Source: CAD feature listing. Evaluate the final solid. Frame: model axes, mm. Face numbers are marked on the shaded views. A direction names the side the tool comes from. Coordinates: 2 decimals unless noted, no trailing zeros. Order: outer loops, then holes, each group sorted by start corner. A loop starts at its lowest first (then second) coordinate and runs counter-clockwise, first axis right, second up.
```python
from build123d import *

# Parameters (mm, degrees)
BOSS_EXTRUDE1_START     = -9
SKETCH1_W               = 152.45
SKETCH1_H               = 16
BOSS_EXTRUDE1_DEPTH     = 5
BOSS_EXTRUDE2_START     = -9
SKETCH2_R               = 6.5
BOSS_EXTRUDE2_DEPTH     = 5
BOSS_EXTRUDE3_START     = -9
SKETCH3_R               = 8
BOSS_EXTRUDE3_DEPTH     = 5
BOSS_EXTRUDE4_START     = -9
SKETCH4_R               = 7
BOSS_EXTRUDE4_DEPTH     = 11.5
BOSS_EXTRUDE5_START     = 2.5
SKETCH5_R               = 5.5
BOSS_EXTRUDE5_DEPTH     = 1
BOSS_EXTRUDE6_START     = -4
SKETCH6_R               = 3.5
BOSS_EXTRUDE6_DEPTH     = 1
CUT_EXTRUDE1_DEPTH      = 132.004589614
CUT_EXTRUDE1_DEPTH_BACK = 132.004589614
SKETCH7_R               = 4
CUT_EXTRUDE2_DEPTH      = 132.004589614
CUT_EXTRUDE2_DEPTH_BACK = 132.004589614
SKETCH8_R               = 1.725
CUT_EXTRUDE3_DEPTH      = 132.004589614
CUT_EXTRUDE3_DEPTH_BACK = 132.004589614
SKETCH9_W               = 22.8
SKETCH9_H               = 11.9
CUT_EXTRUDE4_DEPTH      = 132.004589614
CUT_EXTRUDE4_DEPTH_BACK = 132.004589614
SKETCH10_R              = 0.9


with BuildPart() as part:
    # Sketch1 → Boss-Extrude1 (new body)
    with BuildSketch(Plane.XY.offset(BOSS_EXTRUDE1_START)):
        with Locations((46.225, 0)):
            Rectangle(SKETCH1_W, SKETCH1_H)
    extrude(amount=BOSS_EXTRUDE1_DEPTH)

    # Sketch2 → Boss-Extrude2 (add)
    with BuildSketch(Plane.XY.offset(BOSS_EXTRUDE2_START)):
        with Locations((-30, 0)):
            Circle(SKETCH2_R)
    extrude(amount=BOSS_EXTRUDE2_DEPTH)

    # Sketch3 → Boss-Extrude3 (add)
    with BuildSketch(Plane.XY.offset(BOSS_EXTRUDE3_START)):
        with Locations((122.45, 0)):
            Circle(SKETCH3_R)
    extrude(amount=BOSS_EXTRUDE3_DEPTH)

    # Sketch4 → Boss-Extrude4 (add)
    with BuildSketch(Plane.XY.offset(BOSS_EXTRUDE4_START)):
        Circle(SKETCH4_R)
    extrude(amount=BOSS_EXTRUDE4_DEPTH)

    # Sketch5 → Boss-Extrude5 (add)
    with BuildSketch(Plane.XY.offset(BOSS_EXTRUDE5_START)):
        Circle(SKETCH5_R)
    extrude(amount=BOSS_EXTRUDE5_DEPTH)

    # Sketch6 → Boss-Extrude6 (add)
    with BuildSketch(Plane.XY.offset(BOSS_EXTRUDE6_START)):
        with Locations((-30, 0)):
            Circle(SKETCH6_R)
    extrude(amount=BOSS_EXTRUDE6_DEPTH)

    # Sketch7 → Cut-Extrude1 (cut, two sides: drawn at the far end of the back side and taken through both)
    with BuildSketch(Plane.XY.offset(-CUT_EXTRUDE1_DEPTH_BACK)):
        Circle(SKETCH7_R)
    extrude(amount=CUT_EXTRUDE1_DEPTH + CUT_EXTRUDE1_DEPTH_BACK, mode=Mode.SUBTRACT)

    # Sketch8 → Cut-Extrude2 (cut, two sides: drawn at the far end of the back side and taken through both)
    with BuildSketch(Plane.XY.offset(-CUT_EXTRUDE2_DEPTH_BACK)):
        with Locations((-30, 0)):
            Circle(SKETCH8_R)
    extrude(amount=CUT_EXTRUDE2_DEPTH + CUT_EXTRUDE2_DEPTH_BACK, mode=Mode.SUBTRACT)

    # Sketch9 → Cut-Extrude3 (cut, two sides: drawn at the far end of the back side and taken through both)
    with BuildSketch(Plane.XY.offset(-CUT_EXTRUDE3_DEPTH_BACK)):
        with Locations((114.2, 0)):
            Rectangle(SKETCH9_W, SKETCH9_H)
    extrude(amount=CUT_EXTRUDE3_DEPTH + CUT_EXTRUDE3_DEPTH_BACK, mode=Mode.SUBTRACT)

    # Sketch10 → Cut-Extrude4 (cut, two sides: drawn at the far end of the back side and taken through both)
    with BuildSketch(Plane.XY.offset(-CUT_EXTRUDE4_DEPTH_BACK)):
        with Locations((100.45, 0)):
            Circle(SKETCH10_R)
        with Locations((127.95, 0)):
            Circle(SKETCH10_R)
    extrude(amount=CUT_EXTRUDE4_DEPTH + CUT_EXTRUDE4_DEPTH_BACK, mode=Mode.SUBTRACT)


solid = part.part
```
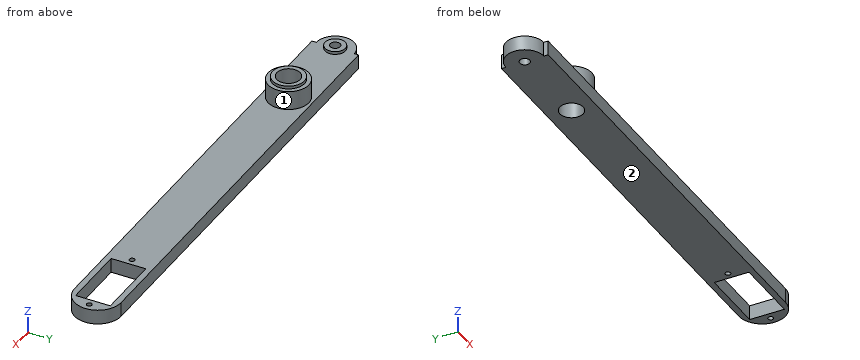
1. Section query C-C on z = 0.75. Return loops of the section in (x, y).
Findings:
outline: circle Ø14 at (0, 0); hole circle Ø8 at (0, 0)
2. Ray query, line 1 (X direction, y = 0, z = -6.2) (3 decimals); line 2 (X direction, y = 0.5, z = -6.5); line 3 (X direction, y = 0, z = 0). Return the intervals inside material, ascending.
Findings:
line 1: x = -36.5 to -31.725, -28.275 to -4, 4 to 99.55, 101.35 to 102.8, 125.6 to 127.05, 128.85 to 130.45
line 2: x = -36.48 to -31.65, -28.35 to -3.97, 3.97 to 99.7, 101.2 to 102.8, 125.6 to 127.2, 128.7 to 130.43
line 3: x = -7 to -4, 4 to 7
3. Access query for the marked faces 1 and 2. Directions: +Z, -Z, +X, -X, +Y, -Y. A direction counts if a zero-diameter tool reaches every point of the face in a straight line with its end or side. Return the directions, or none.
Findings:
face 1: +Z
face 2: -Z, +X, -X, +Y, -Y
4. Section query B-B on x = 0. Return loops of the section in (y, z), plus the area to 3 significant figures.
Findings:
outline: (-8, -9) - (-4, -9) - (-4, 3.5) - (-5.5, 3.5) - (-5.5, 2.5) - (-7, 2.5) - (-7, -4) - (-8, -4) - close; (4, -9) - (8, -9) - (8, -4) - (7, -4) - (7, 2.5) - (5.5, 2.5) - (5.5, 3.5) - (4, 3.5) - close
area: 82.0 mm2
5. Section query A-A on z = -6. Return loops of the section in (x, y) (3 decimals), plus the area to 3 significant figures.
Findings:
outline: (-30, -8) - (122.45, -8) arc R8 ccw to (122.45, 8) - (-30, 8) - (-30, 6.5) arc R6.5 ccw to (-30, -6.5) - close; hole circle Ø3.45 at (-30, 0); hole circle Ø8 at (0, 0); hole circle Ø1.8 at (100.45, 0); hole (102.8, -5.95) - (125.6, -5.95) - (125.6, 5.95) - (102.8, 5.95) - close; hole circle Ø1.8 at (127.95, 0)
area: 2,270 mm2
6. Pin query (flat end, axial travel): P1, Ø1, axis at x = -6, z = -2, coming from the +Y side; P2, Ø2.5, axis at x = 127.95, y = 0, coming from the +Z side; P3, Ø2, axis at x = -31.5, y = 1, coming from the +Z side; P4, Ø4, axis at y = 1, z = -6, coming from the +X side. Return the tip coordinate at first contact, or that it passes through.
Findings:
P1: stops at y = 4.33
P2: stops at z = -4
P3: stops at z = -3
P4: stops at x = 130.45
